```python
from build123d import *

# Parameters (mm, degrees)
F0_R     = 4
F0_R_2   = 8
F1_DEPTH = 6
F2_R     = 5
F3_R     = 3


with BuildPart() as f1:
    # F0 (on Front) → F1 (new body)
    with BuildSketch(Plane.XZ):
        with BuildLine():
            Line((-67.049116, 8.89), (-67.049116, 0))
            Line((-67.049116, 0), (72.650884, 0))
            Line((72.650884, 0), (72.650884, 25.4))
            Line((72.650884, 25.4), (63.910884, 25.4))
            ThreePointArc((63.910884, 25.4), (57.410884, 18.9), (50.910884, 25.4))
            Line((50.910884, 25.4), (-28.949116, 25.4))
            Line((-28.949116, 25.4), (-50.539116, 50.8))
            Line((-50.539116, 50.8), (-67.049116, 50.8))
            Line((-67.049116, 50.8), (-67.049116, 41.91))
            Line((-67.049116, 41.91), (-67.049116, 8.89))
        make_face()
        with Locations((-58.159116, 8.89)):
            Circle(F0_R, mode=Mode.SUBTRACT)
        with Locations((-47.999116, 25.4)):
            Circle(F0_R_2, mode=Mode.SUBTRACT)
        with Locations((63.760884, 8.89)):
            Circle(F0_R, mode=Mode.SUBTRACT)
        with Locations((-58.159116, 41.91)):
            Circle(F0_R, mode=Mode.SUBTRACT)
    extrude(amount=F1_DEPTH)

    # F2
    f2_edges = [f1.edges().sort_by_distance(p)[0] for p in [
        (-67.049116, -3, 50.8),
        (-67.049116, -3, 0),
        (72.650884, -3, 0),
    ]]
    fillet(f2_edges, radius=F2_R)

    # F3
    f3_edges = [f1.edges().sort_by_distance(p)[0] for p in [
        (63.910884, -3, 25.4),
    ]]
    fillet(f3_edges, radius=F3_R)


solid = f1.part
```
For this review, take the finished solid that the model builds, in its own axes (mm). A direction names the side the tool comes from. Round coordinates to 2 decimals unless told otherwise and drop trailing zeros. Write each loop counter-clockwise with the first axis right and the second up, starting at its lowest first coordinate (ties: lowest second). Pieces come first, ordered by that corner, then holes. Notation, with made-up numbers: (29.25, 87.25) -> (47.25, 87.25) arc R21 cw to (47.25, 100.25) -> close; hole circle Ø2 at (-10, 39.5). An arc over 180 degrees is marked (long way). One line per question, with ' | ' between items. Start each with the question number.
(1) Tool access review of faces 4 (the face through (70, -3, 25.4)), 5 (the face through (-56, -3, 50.8)): name each direction out of +Z, -Z, +X, -X, +Y, -Y from which nothing blocks a thin tool from reaching the whole face with its end or side.
(2) Add section D-D, the plane z = 41.91. Write out the cut boundary in (x, y), plus the area to 3 significant figures.
(3) Add section C-C, the plane x = 61.5. Write out the cut boundary in (y, z), plus the area to 3 significant figures.
(4) Mouldability with a two-part tool opening along X and no side actions: class faces 1 (the face through (71.15, -3.04, 1.43)), 2 (the face through (64.69, -3.04, 24.85)), 3 (the face through (-65.62, -3.04, 49.3)) as released by +X, released by -X, zero draft, split by the parting line, or undercut.
(5) For line 1 along Z through (x, y) = (-0.5, -4.85); line 2 along X through (y, z) = (-3.65, 12.5); line 3 along X through (y, z) = (-0.85, 28), list the stretches that pass through material, from the lowest coordinate up. Write a range as from..to.
(6) Add section A-A, the plane z = 8.89. Write out the cut boundary in (x, y).
(7) Insertion check: P1, Ø3, axis at x = 71, y = -3.5, coming from the +Z side; P2, Ø5, axis at x = -58.16, z = 41.91, coming from the +Y side; P3, Ø3, axis at y = -4, z = 40.5, coming from the +X side. Each pin has a flat end and moves straight along its axis. Give the tip position at first contact, or say it passes through.
(8) Add section B-B, the plane y = -1.7. Write out the cut boundary in (x, z), plus the area to 3 significant figures.
Answer list:
1) face 4: +Z, +X, +Y, -Y | face 5: +Z, +X, -X, +Y, -Y
2) outline: (-67.05, -6) -> (-62.16, -6) -> (-62.16, 0) -> (-67.05, 0) -> close; (-54.16, -6) -> (-42.98, -6) -> (-42.98, 0) -> (-54.16, 0) -> close | area: 96.4 mm²
3) outline: (-6, 0) -> (0, 0) -> (0, 5.59) -> (-6, 5.59) -> close; (-6, 12.19) -> (0, 12.19) -> (0, 20.35) -> (-6, 20.35) -> close | area: 82.5 mm²
4) face 1: released by +X | face 2: undercut | face 3: released by -X
5) line 1: 0..25.4 | line 2: -67.05..-59.88, -56.44..62.04, 65.48..72.65 | line 3: -67.05..-55.56, -40.43..-31.16
6) outline: (-67.05, -6) -> (-62.16, -6) -> (-62.16, 0) -> (-67.05, 0) -> close; (-54.16, -6) -> (59.76, -6) -> (59.76, 0) -> (-54.16, 0) -> close; (67.76, -6) -> (72.65, -6) -> (72.65, 0) -> (67.76, 0) -> close
7) P1: z = 25.4 | P2: through | P3: x = -40.51
8) outline: (-67.05, 5) arc R5 ccw to (-62.05, 0) -> (67.65, 0) arc R5 ccw to (72.65, 5) -> (72.65, 25.4) -> (66.42, 25.4) arc R3 ccw to (63.58, 23.35) arc R6.5 cw to (50.91, 25.4) -> (-28.95, 25.4) -> (-50.54, 50.8) -> (-62.05, 50.8) arc R5 ccw to (-67.05, 45.8) -> close; hole circle Ø8 at (-58.16, 8.89); hole circle Ø8 at (-58.16, 41.91); hole circle Ø16 at (-48, 25.4); hole circle Ø8 at (63.76, 8.89) | area: 3,810 mm²
